The listing builds one solid part. Answer for the finished solid, in the listing's coordinates (mm). Coordinates: 2 decimals unless noted, no trailing zeros. Write each loop counter-clockwise with the first axis right and the second up, starting at its lowest first coordinate (ties: lowest second). Pieces come first, ordered by that corner, then holes.
from build123d import *

# Parameters (mm, degrees)
F0_W     = 300
F0_H     = 100
F1_DEPTH = 50
F2_R     = 49.99999
F3_R     = 25
F4_DEPTH = 50


# Not quite as in the source:
# - a fillet or chamfer is up to 0.001 mm smaller than in the source, because OpenCascade refuses the exact size


with BuildPart() as f1:
    # F0 (on Right) → F1 (new body)
    with BuildSketch(Plane.YZ):
        Rectangle(F0_W, F0_H)
    extrude(amount=F1_DEPTH)

    # F2 (radius 50 in the source; OpenCascade refuses exactly that, so slightly less here)
    f2_edges = [f1.edges().sort_by_distance(p)[0] for p in [
        (25, -150, 50),
        (25, -150, -50),
        (25, 150, 50),
        (25, 150, -50),
    ]]
    fillet(f2_edges, radius=F2_R)

    # F3 (on face) → F4 (cut)
    with BuildSketch(Plane.YZ.offset(50)):
        with Locations((-100, 0)):
            Circle(F3_R)
        with Locations((100, 0)):
            Circle(F3_R)
    extrude(amount=-F4_DEPTH, mode=Mode.SUBTRACT)


solid = f1.part
Q1. Given pin 1 (1.5 mm diameter, centred on x = 10.5, z = -24.5, fed in from +Y); pin 2 (2 mm diameter, centred on x = 23.5, z = 32, fed in from +Y); pin 3 (2 mm diameter, centred on x = 23.5, z = -8.5, fed in from +Y), each flat-ended and moving along its own axis, determine where each tip first touches the part or whether it passes through.
Answers below:
pin 1: stops at y = 144
pin 2: stops at y = 139.23
pin 3: stops at y = 149.43
Q2. The part is cut by section D-D, the plane z = -21. Write down the section's boundary in (x, y), then the cut area to 3 significant figures.
Answers below:
outline: (0, -145.38) - (50, -145.38) - (50, -113.56) - (0, -113.56) - close; (0, -86.44) - (50, -86.44) - (50, 86.44) - (0, 86.44) - close; (0, 113.56) - (50, 113.56) - (50, 145.38) - (0, 145.38) - close
area: 11,800 mm2
Q3. The part is cut by section B-B, the plane z = 15. Write down the section's boundary in (x, y), then the cut area to 3 significant figures.
Answers below:
outline: (0, -147.7) - (50, -147.7) - (50, -120) - (0, -120) - close; (0, -80) - (50, -80) - (50, 80) - (0, 80) - close; (0, 120) - (50, 120) - (50, 147.7) - (0, 147.7) - close
area: 10,800 mm2
Q4. The part is cut by section C-C, the plane y = -119. Write down the section's boundary in (x, z), then the cut area to 3 significant figures.
Answers below:
outline: (0, -46.25) - (50, -46.25) - (50, -16.25) - (0, -16.25) - close; (0, 16.25) - (50, 16.25) - (50, 46.25) - (0, 46.25) - close
area: 3,000 mm2
Q5. Determine the mould class of faces 1 (the face through (25.35, 75.024, 1.099)), 2 (the face through (25.35, -135.742, 34.964)), 3 (the face through (25, -1, -50)) for opening direction Z: released by +Z, released by -Z, zero draft, split by the parting line, or undercut.
Answers below:
face 1: undercut
face 2: released by +Z
face 3: released by -Z
Q6. The part is cut by section A-A, the plane x = 36. State how many separate pieces and enclosed holes the cut face has, then the cut area to 3 significant figures.
Answers below:
separate pieces: 1
enclosed holes: 2
area: 23,900 mm2
Q7. Find the intervals of material crossed by probe 1 along Y at (x, z) = (42.5, -1.5); probe 2 along Y at (x, z) = (20, -5); probe 3 along Z at (x, y) = (24, -100), in increasing order.
Answers below:
probe 1: y = -149.98 to -124.95, -75.05 to 75.05, 124.95 to 149.98
probe 2: y = -149.75 to -124.49, -75.51 to 75.51, 124.49 to 149.75
probe 3: z = -50 to -25, 25 to 50
